```python
from build123d import *

# Parameters (mm, degrees)
EXTRUDE_1_DEPTH     = 6
SKETCH_2_R          = 25
EXTRUDE_2_DEPTH     = 9.5
SKETCH_3_R          = 20
CUT_EXTRUDE_1_DEPTH = 12
SKETCH_4_R          = 15
CUT_EXTRUDE_2_DEPTH = 79.70196948
HOLE_WIZARD_1_D     = 8.5
HOLE_WIZARD_1_DEPTH = 93.98
HOLE_WIZARD_M8_1_D  = 6.8


with BuildPart() as part:
    # 草图1 → 凸台-拉伸1 (new body)
    with BuildSketch(Plane.XY):
        with BuildLine():
            Line((21.426473245, 32), (-21.426473245, 32))
            ThreePointArc((-21.426473245, 32), (-23.263590552, 32.628291755), (-24.331210755, 34.25))
            ThreePointArc((-24.331210755, 34.25), (-30.746282552, 40.701376437), (-39.510832187, 38.260869565))
            ThreePointArc((-39.510832187, 38.260869565), (0, -55), (39.510832187, 38.260869565))
            ThreePointArc((39.510832187, 38.260869565), (30.746282552, 40.701376437), (24.331210755, 34.25))
            ThreePointArc((24.331210755, 34.25), (23.263590552, 32.628291755), (21.426473245, 32))
        make_face()
    extrude(amount=EXTRUDE_1_DEPTH)

    # 草图2 → 凸台-拉伸2 (add)
    with BuildSketch(Plane.XY.offset(6)):
        with Locations(Location((0, 0, 0), (0, 0, 180))):
            Circle(SKETCH_2_R)
    extrude(amount=EXTRUDE_2_DEPTH)

    # 草图3 → 切除-拉伸1 (cut)
    with BuildSketch(Plane(origin=(0, 0, 0), x_dir=(-1, 0, 0), z_dir=(0, 0, -1))):
        Circle(SKETCH_3_R)
    extrude(amount=-CUT_EXTRUDE_1_DEPTH, mode=Mode.SUBTRACT)

    # 草图4 → 切除-拉伸2 (cut, through all)
    with BuildSketch(Plane(origin=(0, 0, 12), x_dir=(-1, 0, 0), z_dir=(0, 0, -1))):
        Circle(SKETCH_4_R)
    extrude(amount=-CUT_EXTRUDE_2_DEPTH, mode=Mode.SUBTRACT)

    # 孔1
    with Locations(Plane.XY.offset(6)):
        with Locations((33.045423284, 32), (0, -46)):
            Hole(HOLE_WIZARD_1_D / 2, depth=HOLE_WIZARD_1_DEPTH)

    # M8 螺纹孔1 (through all)
    with Locations(Plane.XY.offset(6)):
        with Locations((46, 0), (-46, 0)):
            Hole(HOLE_WIZARD_M8_1_D / 2)

    # 草图11 → Ø8.5 (8.5) 直径孔1 (revolve, cut)
    with BuildSketch(Plane(origin=(-33.045423284, 32, 6), x_dir=(0, -1, 0), z_dir=(1, 0, 0))):
        Polygon((0, 0), (0, 6), (4.25, 6), (4.25, 2.25), (6.5, 0), align=None)
    revolve(axis=Axis((-33.045423284, 32, 12.35), (0, 0, -1)), mode=Mode.SUBTRACT)


solid = part.part
```
Check sheet for the modelled part. Datum: model origin and axes. Units: mm. A direction names the side the tool comes from. Give positions to 0.01 mm unless a question says otherwise; leave off trailing zeros. Order: outer loops, then holes, each group sorted by start corner. A loop starts at its lowest first (then second) coordinate and runs counter-clockwise, first axis right, second up. Notation, with made-up numbers: (65.5, 89) -> (71.5, 89) arc R28 cw to (71.5, 125) -> close; hole circle Ø6 at (46, -23). An arc over 180 degrees is marked (long way). Use CSV: the item, a comma, the result in double quotes. Start each with the question number.
1) Mould release check, pull along X, two halves, no side actions. Record for faces 1 (the face through (30.876, 40.735, 2.958)), 2 (the face through (-23.846, -7.509, 10.683)), 3 (the face through (-1, -28, 6)): released by +X, released by -X, zero draft, split by the parting line, or undercut.
2) Material ranges on line 1 (Y direction, x = 0, z = 5.5); line 2 (Y direction, x = 0, z = 14.05); line 3 (Z direction, x = -27, y = -31), recorded low to high. Write a range as from..to.
3) Sectioned sample at C-C, the plane y = -13. Record the boundary of the cut face in (x, z), plus the area to 3 significant figures.
4) Go/stop test with flat-tipped pins: P1, Ø6, axis at x = 46, y = 0, coming from the +Z side; P2, Ø10, axis at x = -33.05, y = 32, coming from the +Z side; P3, Ø1, axis at y = 14, z = 7, coming from the -X side; P4, Ø6.5, axis at x = 2, z = 3.5, coming from the +Y side. Record where each tip stops, or that it passes through.
5) Sectioned sample at D-D, the plane z = 2.5. Record the boundary of the cut face in (x, y), plus the area to 3 significant figures.
6) Set-up check for faces 4 (the face through (-23.24, 32.61, 2.96)), 5 (the face through (-3, 15, 12)), 6 (the face through (29.12, 30.37, 2.96)): record each of +Z, -Z, +X, -X, +Y, -Y from which the full face is reachable in a straight line by a thin tool's end or side.
7) Sectioned sample at A-A, the plane y = 0. Record the boundary of the cut face in (x, z), plus the area to 3 significant figures.
8) Sectioned sample at B-B, the plane x = -46. Record the boundary of the cut face in (y, z), plus the area to 3 significant figures.
Recorded:
1,face 1,"undercut"
1,face 2,"split by the parting line"
1,face 3,"zero draft"
2,line 1,"-55..-50.25, -41.75..-20, 20..32"
2,line 2,"-25..-15, 15..25"
2,line 3,"0..6"
3,outline,"(-53.44, 0) -> (-15.2, 0) -> (-15.2, 12) -> (-7.48, 12) -> (-7.48, 15.5) -> (-21.35, 15.5) -> (-21.35, 6) -> (-53.44, 6) -> close; (7.48, 12) -> (15.2, 12) -> (15.2, 0) -> (53.44, 0) -> (53.44, 6) -> (21.35, 6) -> (21.35, 15.5) -> (7.48, 15.5) -> close"
3,area,"630 mm2"
4,P1,"through"
4,P2,"z = 4.5"
4,P3,"x = -21.04"
4,P4,"y = 32"
5,outline,"(-39.51, 38.26) arc R55 ccw (long way) to (39.51, 38.26) arc R9 ccw to (24.33, 34.25) arc R3 cw to (21.43, 32) -> (-21.43, 32) arc R3 cw to (-24.33, 34.25) arc R9 ccw to start; hole circle Ø6.8 at (-46, 0); hole circle Ø8.5 at (-33.05, 32); hole circle Ø40 at (0, 0); hole circle Ø8.5 at (0, -46); hole circle Ø8.5 at (33.05, 32); hole circle Ø6.8 at (46, 0)"
5,area,"6,830 mm2"
6,face 4,"+Z, -Z, +Y"
6,face 5,"-Z"
6,face 6,"+Z, -Z"
7,outline,"(-55, 0) -> (-49.4, 0) -> (-49.4, 6) -> (-55, 6) -> close; (-42.6, 0) -> (-20, 0) -> (-20, 12) -> (-15, 12) -> (-15, 15.5) -> (-25, 15.5) -> (-25, 6) -> (-42.6, 6) -> close; (15, 12) -> (20, 12) -> (20, 0) -> (42.6, 0) -> (42.6, 6) -> (25, 6) -> (25, 15.5) -> (15, 15.5) -> close; (49.4, 0) -> (55, 0) -> (55, 6) -> (49.4, 6) -> close"
7,area,"468 mm2"
8,outline,"(-30.15, 0) -> (-3.4, 0) -> (-3.4, 6) -> (-30.15, 6) -> close; (3.4, 0) -> (30.15, 0) -> (30.15, 6) -> (3.4, 6) -> close"
8,area,"321 mm2"
